Geometry: final body of the model. Coordinates: model frame, mm. Face numbers are marked on the shaded views. A direction names the side the tool comes from. Give positions to 0.01 mm unless a question says otherwise; leave off trailing zeros. Write each loop counter-clockwise with the first axis right and the second up, starting at its lowest first coordinate (ties: lowest second). Pieces come first, ordered by that corner, then holes. Notation, with made-up numbers: M 60,-4 L 119,-4 A7 cw 119,8 Z; hole C 70,89.25 d4. An arc over 180 degrees is marked long. Use a Markdown table: item, result. Add a question column.
1) Pin query (flat end, axial travel): pin 1 (12 mm diameter, centred on y = 4.5, z = 43, fed in from -X); pin 2 (12 mm diameter, centred on x = 0.5, z = 80.5, fed in from +Y); pin 3 (12 mm diameter, centred on x = 5.5, z = 117.5, fed in from -Y). Return the tip coordinate at first contact, or that it passes through.
2) Line query: line 1 (Y direction, x = -1, z = 89); line 2 (Z direction, x = -14, y = -10); line 3 (X direction, y = -21, z = 15). Output: solid intervals per line, ascending.
3) Section B-B on y = -20. Return the cut outline in (x, z).
4) Section C-C on x = 17.5. Return the cut outline in (y, z).
5) Set-up query: the marked faces 1 and 2. Return all of +Z, -Z, +X, -X, +Y, -Y with unobstructed straight access to the full face (end or side cutting, diameter ignored); none if empty.
6) Section A-A on z = 29. Return the cut outline in (x, y), then the cut area to 3 significant figures.
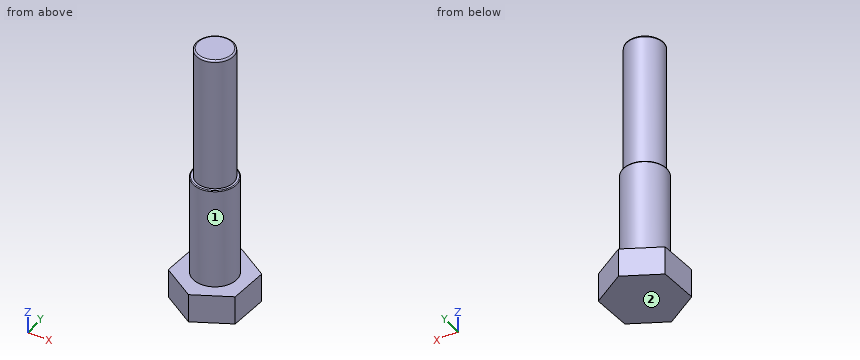
```python
from build123d import *

# Parameters (mm, degrees)
EXTRUDE_276_DEPTH = 17
SKETCH_2_R        = 12.9
EXTRUDE_1_DEPTH   = 60
SKETCH_3_R        = 11
EXTRUDE_2_DEPTH   = 80
FILLET_2_R        = 1
FILLET_4_R        = 0.5


with BuildPart() as part:
    # 草图1 → Extrude 276 (new body)
    with BuildSketch(Plane.XY):
        Polygon((20.984201837, 10.954296262), (1.005402075, 23.65), (-19.978799762, 12.695703738), (-20.984201837, -10.954296262), (-1.005402075, -23.65), (19.978799762, -12.695703738), align=None)
    extrude(amount=EXTRUDE_276_DEPTH)

    # 草图2 → 凸台-拉伸1 (add)
    with BuildSketch(Plane.XY.offset(17)):
        with Locations(Location((0, 0, 0), (0, 0, 180))):
            Circle(SKETCH_2_R)
    extrude(amount=EXTRUDE_1_DEPTH)

    # 草图3 → 凸台-拉伸2 (add)
    with BuildSketch(Plane.XY.offset(77)):
        Circle(SKETCH_3_R)
    extrude(amount=EXTRUDE_2_DEPTH)

    # 圆角2
    fillet_2_edges = [part.edges().sort_by_distance(p)[0] for p in [
        (-11, 0, 157),
    ]]
    fillet(fillet_2_edges, radius=FILLET_2_R)

    # 圆角4
    fillet_4_edges = [part.edges().sort_by_distance(p)[0] for p in [
        (12.9, 0, 77),
    ]]
    fillet(fillet_4_edges, radius=FILLET_4_R)


solid = part.part
```
Found:
| question | item | result |
|---|---|---|
| 1 | pin 1 | x = -12.9 |
| 1 | pin 2 | y = 12.9 |
| 1 | pin 3 | y = -11 |
| 2 | line 1 | -10.95 to 10.95 |
| 2 | line 2 | 0 to 17 |
| 2 | line 3 | -5.18 to 4.07 |
| 3 | outline | M -6.75,0 L 5.99,0 L 5.99,17 L -6.75,17 Z |
| 4 | outline | M -13.99,0 L 13.17,0 L 13.17,17 L -13.99,17 Z |
| 5 | face 1 | +Z |
| 5 | face 2 | -Z, +X, -X, +Y, -Y |
| 6 | outline | C 0,0 d25.8 |
| 6 | area | 523 mm² |
